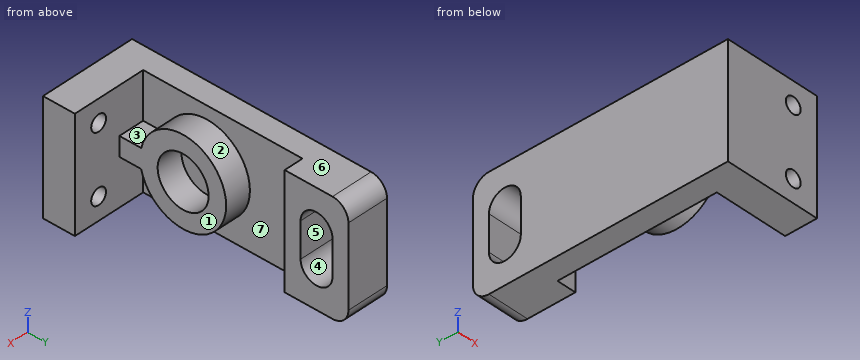
from build123d import *

# Parameters (mm, degrees)
IZIM1_W                     = 30
IZIM1_H                     = 35
Y_KSEKLIK_EKSTR_ZYON1_DEPTH = 10
IZIM2_W                     = 7
IZIM2_H                     = 35
Y_KSEKLIK_EKSTR_ZYON2_DEPTH = 70
IZIM3_W                     = 35
IZIM3_H                     = 20
Y_KSEKLIK_EKSTR_ZYON3_DEPTH = 6
RADYUS1_R                   = 5
KES_EKSTR_ZYON1_DEPTH       = 14
IZIM5_R                     = 2.5
KES_EKSTR_ZYON2_DEPTH       = 11
IZIM6_R                     = 8
Y_KSEKLIK_EKSTR_ZYON4_DEPTH = 8


with BuildPart() as part:
    # Çizim1 → Yükseklik-Ekstrüzyon1 (new body)
    with BuildSketch(Plane(origin=(0, 0, 0), x_dir=(1, 0, 0), z_dir=(0, 1, 0))):
        Rectangle(IZIM1_W, IZIM1_H)
    extrude(amount=Y_KSEKLIK_EKSTR_ZYON1_DEPTH)

    # Çizim2 → Yükseklik-Ekstrüzyon2 (add)
    with BuildSketch(Plane(origin=(0, 10, 0), x_dir=(1, 0, 0), z_dir=(0, 1, 0))):
        with Locations((-11.5, 0)):
            Rectangle(IZIM2_W, IZIM2_H)
    extrude(amount=Y_KSEKLIK_EKSTR_ZYON2_DEPTH)

    # Çizim3 → Yükseklik-Ekstrüzyon3 (add)
    with BuildSketch(Plane(origin=(-8, 0, 0), x_dir=(0, 0, -1), z_dir=(1, 0, 0))):
        with Locations((0, 70)):
            Rectangle(IZIM3_W, IZIM3_H)
    extrude(amount=Y_KSEKLIK_EKSTR_ZYON3_DEPTH)

    # Radyus1
    radyus1_edges = [part.edges().sort_by_distance(p)[0] for p in [
        (-8.5, 80, 17.5),
        (-8.5, 80, -17.5),
    ]]
    fillet(radyus1_edges, radius=RADYUS1_R)

    # Çizim4 → Kes-Ekstrüzyon1 (cut, through all)
    with BuildSketch(Plane(origin=(-2, 0, 0), x_dir=(0, 0, -1), z_dir=(1, 0, 0))):
        with BuildLine():
            Line((-5.5, 75), (5.5, 75))
            ThreePointArc((5.5, 75), (10.5, 70), (5.5, 65))
            Line((5.5, 65), (-5.5, 65))
            ThreePointArc((-5.5, 65), (-10.5, 70), (-5.5, 75))
        make_face()
    extrude(amount=-KES_EKSTR_ZYON1_DEPTH, mode=Mode.SUBTRACT)

    # Çizim5 → Kes-Ekstrüzyon2 (cut, through all)
    with BuildSketch(Plane(origin=(0, 10, 0), x_dir=(1, 0, 0), z_dir=(0, 1, 0))):
        with Locations((7, 10.5)):
            Circle(IZIM5_R)
        with Locations((7, -10.5)):
            Circle(IZIM5_R)
    extrude(amount=-KES_EKSTR_ZYON2_DEPTH, mode=Mode.SUBTRACT)

    # Çizim6 → Yükseklik-Ekstrüzyon4 (add)
    with BuildSketch(Plane(origin=(-8, 0, 0), x_dir=(0, 0, -1), z_dir=(1, 0, 0))):
        with BuildLine():
            Line((-3, 10), (3, 10))
            Line((3, 10), (3, 16.837553419))
            ThreePointArc((3, 16.837553419), (0, 43.5), (-3, 16.837553419))
            Line((-3, 16.837553419), (-3, 10))
        make_face()
        with Locations((0, 30)):
            Circle(IZIM6_R, mode=Mode.SUBTRACT)
    extrude(amount=Y_KSEKLIK_EKSTR_ZYON4_DEPTH)


solid = part.part
Can you work these out from the model? Positions are in its coordinate system, mm. Face numbers are marked on the shaded views. A direction names the side the tool comes from. Coordinates: 2 decimals unless noted, no trailing zeros. Write each loop counter-clockwise with the first axis right and the second up, starting at its lowest first coordinate (ties: lowest second). Pieces come first, ordered by that corner, then holes. Notation, with made-up numbers: (49, 8.25) -> (95, 8.25) arc R21 ccw to (95, 42.25) -> close; hole circle Ø3 at (41, -30). An arc over 180 degrees is marked (long way). Write item = value, one per line.
(1) Imagine slicing it at A-A (x = -6.5). Please give me the cut outline in (y, z), and give its area (3 significant figures).
Verdict:
outline = (0, -17.5) -> (10, -17.5) -> (10, -3) -> (16.84, -3) arc R13.5 ccw (long way) to (16.84, 3) -> (10, 3) -> (10, 17.5) -> (0, 17.5) -> close; (60, -17.5) -> (75, -17.5) arc R5 ccw to (80, -12.5) -> (80, 12.5) arc R5 ccw to (75, 17.5) -> (60, 17.5) -> close; hole circle Ø16 at (30, 0); hole (65, -5.5) arc R5 ccw to (75, -5.5) -> (75, 5.5) arc R5 ccw to (65, 5.5) -> close
area = 1,260 mm^2
(2) For pin 1 (7 mm diameter, centred on x = 5.5, z = 0, fed in from +Y); pin 2 (10 mm diameter, centred on y = 73, z = 8.5, fed in from +X); pin 3 (8 mm diameter, centred on y = 27, z = 0.5, fed in from +X); pin 4 (3 mm diameter, centred on x = 7, z = -10.5, fed in from -Y), each with a flat end and sliding along its axis, tell me the tip position at first contact or that it passes through.
Verdict:
pin_1 = 10
pin_2 = -2
pin_3 = -8
pin_4 = through
(3) On a 3-axis mill with a long thin cutter (end or side, diameter ignored), from which of +Z, -Z, +X, -X, +Y, -Y can I reach the whole of each face in a straight line? I mean the marked faces 1, 2, 3 and 4. Say none if no direction works.
Verdict:
face_1 = +Z, -Z, +X, +Y
face_2 = +X
face_3 = +Z, +X
face_4 = +X, -X
(4) Thinking about a two-plate mould opening in Z: for the marked faces 5, 6 and 7, which applies, +Z half, -Z half, draft (parallel to the pull), parting line (faces both ways), or undercut?
Verdict:
face_5 = undercut
face_6 = +Z half
face_7 = draft
(5) Imagine slicing it at C-C (y = 30). Please give me the cut outline in (x, z), and give its area (3 significant figures).
Verdict:
outline = (-15, -17.5) -> (-8, -17.5) -> (-8, -13.5) -> (0, -13.5) -> (0, -8) -> (-8, -8) -> (-8, 8) -> (0, 8) -> (0, 13.5) -> (-8, 13.5) -> (-8, 17.5) -> (-15, 17.5) -> close
area = 333 mm^2
(6) Imagine slicing it at B-B (z = 0). Please give me the cut outline in (x, y).
Verdict:
outline = (-15, 0) -> (15, 0) -> (15, 10) -> (0, 10) -> (0, 22) -> (-8, 22) -> (-8, 38) -> (0, 38) -> (0, 43.5) -> (-8, 43.5) -> (-8, 60) -> (-2, 60) -> (-2, 65) -> (-15, 65) -> close; (-15, 75) -> (-2, 75) -> (-2, 80) -> (-15, 80) -> close
(7) Imagine slicing it at D-D (z = -11.5). Please give me the cut outline in (x, y).
Verdict:
outline = (-15, 0) -> (4.71, 0) -> (4.71, 10) -> (-8, 10) -> (-8, 22.93) -> (0, 22.93) -> (0, 37.07) -> (-8, 37.07) -> (-8, 60) -> (-2, 60) -> (-2, 80) -> (-15, 80) -> close; (9.29, 0) -> (15, 0) -> (15, 10) -> (9.29, 10) -> close
(8) If I drill on probe 1 along Z at (x, y) = (7, 4.25); probe 2 along X at (y, z) = (3, -10.5); probe 3 along Y at (x, z) = (-5.25, 11), over which ranges is the centre line in solid material (lowest first)?
Verdict:
probe_1 = -17.5 to -13, -8 to 8, 13 to 17.5
probe_2 = -15 to 4.5, 9.5 to 15
probe_3 = 0 to 10, 22.17 to 37.83, 60 to 80
